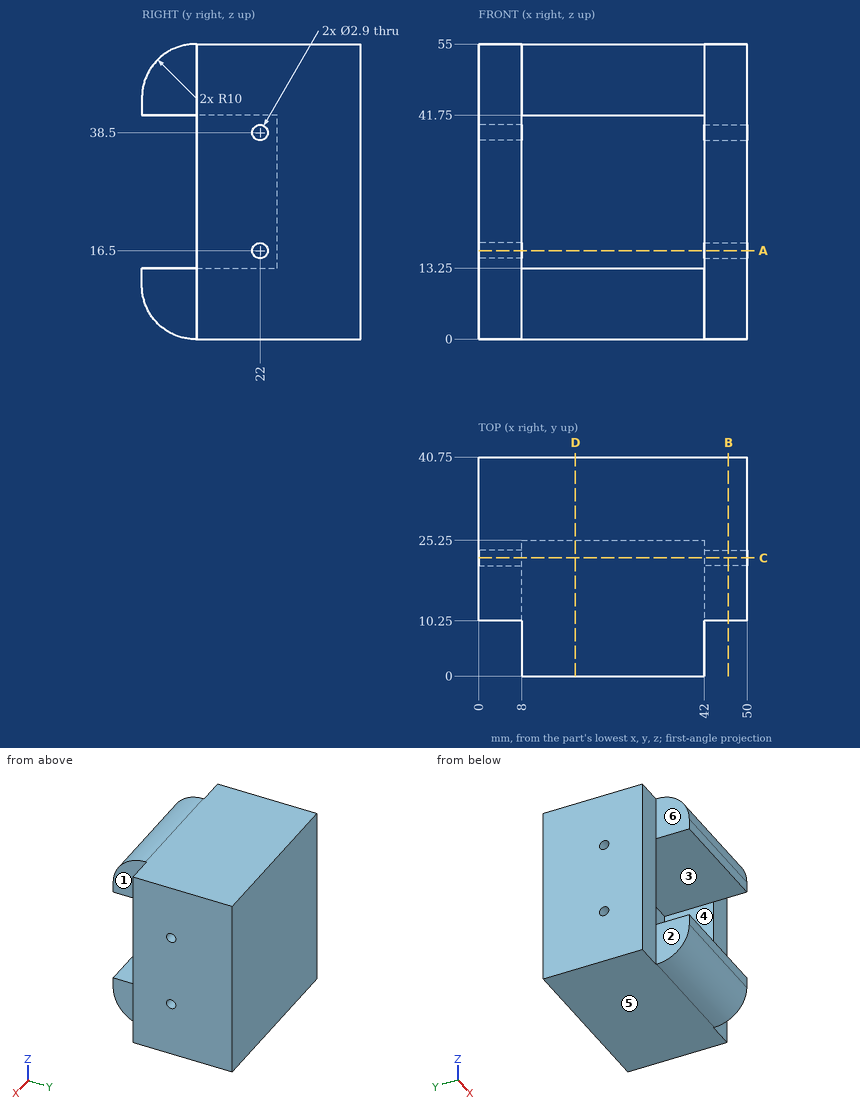
Study the drawing (mm; zero at the part's minimum x, y, z) and answer. A direction names the side the tool comes from. Coordinates: 2 decimals unless noted, no trailing zeros. Write each loop counter-clockwise with the first axis right and the second up, starting at its lowest first coordinate (ties: lowest second). Pieces come first, ordered by that corner, then holes.
Q1. A cutting plane is placed at D-D, the plane x = 18. Give the vertices of the cut face in (y, z), then the cut area to 3 significant figures.
Q2. Which of the six approach directions +Z, -Z, +X, -X, +Y, -Y give full straight-line access (tool end or side, diameter ignored) to the marked faces 1, 2 and 3?
Q3. A cutting plane is placed at B-B, the plane x = 46.5. Give the vertices of the cut face in (y, z), then the cut area to 3 significant figures.
Q4. Each of these flat-tipped pins is pushed along its axis until it touches: pin 1 Ø8 at (y, z) = (5.5, 50.5) entering from -X; pin 2 Ø6.5 at (x, z) = (2.5, 41) entering from -Y; pin 3 Ø5 at (y, z) = (4, 45) entering from +X. Where does it stop, or does it pass through?
Q5. A cutting plane is placed at C-C, the plane y = 22. Give the vertices of the cut face in (x, z), then the cut area to 3 significant figures.
Q6. Determine the mould class of the marked faces 4, 5 and 6 for opening direction X: released by +X, released by -X, zero draft, split by the parting line, or undercut.
Q7. A cutting plane is placed at A-A, the plane z = 16.5. Give the vertices of the cut face in (x, y).
Q8. Find the intervals of material crossed by line 1 (Z direction, x = 3, y = 22); line 2 (X direction, y = 22.5, z = 26); line 3 (Y direction, x = 22.5, z = 28.5), in increasing order.
Findings below:
1. outline: (0, 10) arc R10 ccw to (10, 0) - (40.75, 0) - (40.75, 55) - (10, 55) arc R10 ccw to (0, 45) - (0, 41.75) - (25.25, 41.75) - (25.25, 13.25) - (0, 13.25) - close
1. area: 1,480 mm2
2. face 1: +Z, -Z, +X, -Y
2. face 2: +Z, -Z, -X, -Y
2. face 3: -Y
3. outline: (10.25, 0) - (40.75, 0) - (40.75, 55) - (10.25, 55) - close; hole circle Ø2.9 at (22, 16.5); hole circle Ø2.9 at (22, 38.5)
3. area: 1,660 mm2
4. pin 1: stops at x = 8
4. pin 2: stops at y = 10.25
4. pin 3: stops at x = 42
5. outline: (0, 0) - (50, 0) - (50, 15.05) - (42, 15.05) - (42, 13.25) - (8, 13.25) - (8, 15.05) - (0, 15.05) - close; (0, 17.95) - (8, 17.95) - (8, 37.05) - (0, 37.05) - close; (0, 39.95) - (8, 39.95) - (8, 41.75) - (42, 41.75) - (42, 39.95) - (50, 39.95) - (50, 55) - (0, 55) - close; (42, 17.95) - (50, 17.95) - (50, 37.05) - (42, 37.05) - close
5. area: 1,690 mm2
6. face 4: undercut
6. face 5: zero draft
6. face 6: released by -X
7. outline: (0, 10.25) - (8, 10.25) - (8, 20.55) - (0, 20.55) - close; (0, 23.45) - (8, 23.45) - (8, 25.25) - (42, 25.25) - (42, 23.45) - (50, 23.45) - (50, 40.75) - (0, 40.75) - close; (42, 10.25) - (50, 10.25) - (50, 20.55) - (42, 20.55) - close
8. line 1: z = 0 to 15.05, 17.95 to 37.05, 39.95 to 55
8. line 2: x = 0 to 8, 42 to 50
8. line 3: y = 25.25 to 40.75
